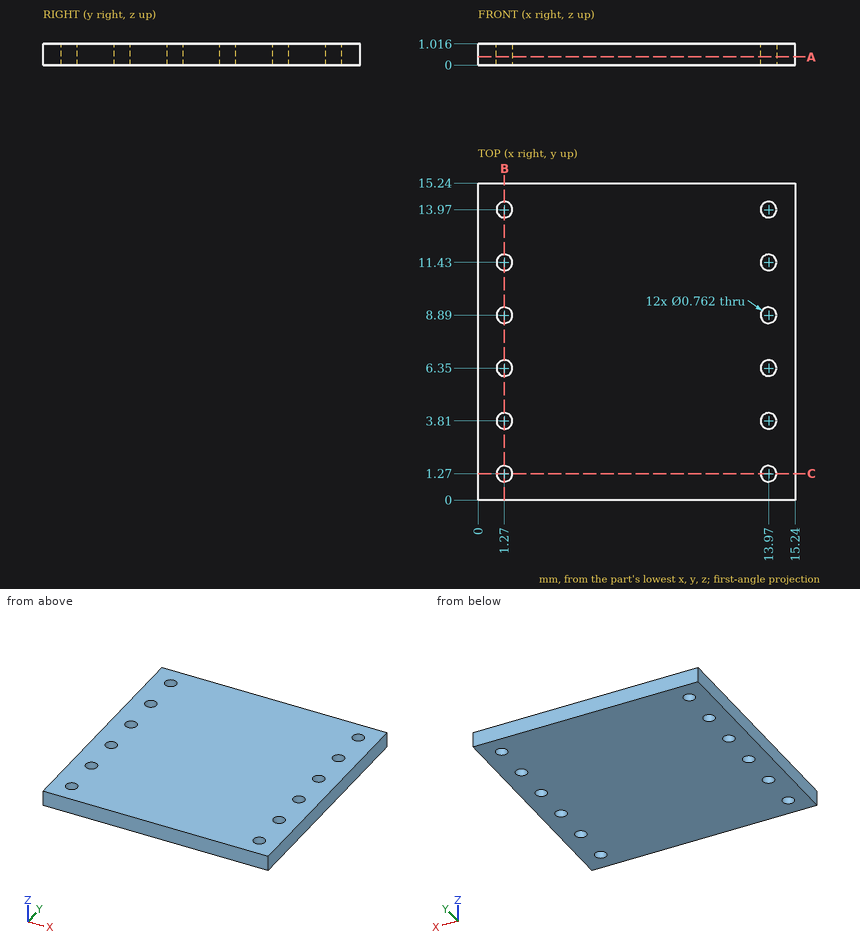
Geometry check sheet. Reference: drawing and pictorial views, mm from the part's lowest x, y, z. Round coordinates to 2 decimals unless told otherwise and drop trailing zeros. Loops run counter-clockwise (first coordinate to the right, second up) from the corner with the lowest first, then second, coordinate; pieces in that order, holes last. Notation, with made-up numbers: (4.5, 58.25) - (51.5, 58.25) arc R11 ccw to (51.5, 79.25) - close; hole circle Ø10 at (-17.75, 21). An arc over 180 degrees is marked (long way). Use a Markdown table: item, result. Add a question column.
1. Thickness scan on probe 1 along X at (y, z) = (6.5, 0.7). Record the ranges inside material, lowest first. Write a range as [from, to].
2. Section check C-C, the plane y = 1.27. Record the boundary of the cut face in (x, z), plus the area to 3 significant figures.
3. Section check A-A, the plane z = 0.4. Give the number of separate pieces and of enclosed holes in the cut face, plus the area to 3 significant figures.
4. Section check B-B, the plane x = 1.27. Record the boundary of the cut face in (y, z), plus the area to 3 significant figures.
Checks:
| question | item | result |
|---|---|---|
| 1 | probe 1 | x = [0, 0.92], [1.62, 13.62], [14.32, 15.24] |
| 2 | outline | (0, 0) - (0.89, 0) - (0.89, 1.02) - (0, 1.02) - close; (1.65, 0) - (13.59, 0) - (13.59, 1.02) - (1.65, 1.02) - close; (14.35, 0) - (15.24, 0) - (15.24, 1.02) - (14.35, 1.02) - close |
| 2 | area | 13.9 mm^2 |
| 3 | separate pieces | 1 |
| 3 | enclosed holes | 12 |
| 3 | area | 227 mm^2 |
| 4 | outline | (0, 0) - (0.89, 0) - (0.89, 1.02) - (0, 1.02) - close; (1.65, 0) - (3.43, 0) - (3.43, 1.02) - (1.65, 1.02) - close; (4.19, 0) - (5.97, 0) - (5.97, 1.02) - (4.19, 1.02) - close; (6.73, 0) - (8.51, 0) - (8.51, 1.02) - (6.73, 1.02) - close; (9.27, 0) - (11.05, 0) - (11.05, 1.02) - (9.27, 1.02) - close; (11.81, 0) - (13.59, 0) - (13.59, 1.02) - (11.81, 1.02) - close; (14.35, 0) - (15.24, 0) - (15.24, 1.02) - (14.35, 1.02) - close |
| 4 | area | 10.8 mm^2 |
